Read the model definition and answer for the solid it produces. Units are mm, in the model's axes. A direction names the side the tool comes from. Round coordinates to 2 decimals unless told otherwise and drop trailing zeros. Write each loop counter-clockwise with the first axis right and the second up, starting at its lowest first coordinate (ties: lowest second). Pieces come first, ordered by that corner, then holes.
from build123d import *

# Parameters (mm, degrees)
F1_DEPTH       = 12.5
F2_R           = 5
F4_D           = 5
F4_DEPTH       = 20
F4_CBORE_D     = 10
F4_CBORE_DEPTH = 5
F4_TIP         = 1.5021515476
F6_D           = 4
F6_CSINK_D     = 10
F6_CSINK_ANGLE = 90


with BuildPart() as f1:
    # F0 (on Top) → F1 (new body, symmetric)
    with BuildSketch(Plane.XY):
        with BuildLine():
            Line((75, 27.5), (-75, 27.5))
            Line((-75, 27.5), (-75, -27.5))
            Line((-75, -27.5), (-25, -27.5))
            ThreePointArc((-25, -27.5), (0, -2.5), (25, -27.5))
            Line((25, -27.5), (75, -27.5))
            Line((75, -27.5), (75, 27.5))
        make_face()
    extrude(amount=F1_DEPTH, both=True)

    # F2
    f2_edges = [f1.edges().sort_by_distance(p)[0] for p in [
        (75, 27.5, 0),
        (-75, 27.5, 0),
        (-75, -27.5, 0),
        (75, -27.5, 0),
    ]]
    fillet(f2_edges, radius=F2_R)

    # F4
    with Locations(Plane.XY.offset(12.5)):
        with Locations((-55, 7.5), (55, 7.5)):
            CounterBoreHole(F4_D / 2, F4_CBORE_D / 2, F4_CBORE_DEPTH, depth=F4_DEPTH)
            with Locations((0, 0, -(F4_DEPTH + F4_TIP / 2))):  # 118° drill point
                Cone(0, F4_D / 2, F4_TIP, mode=Mode.SUBTRACT)

    # F6 (through all)
    with Locations(Plane(origin=(0, 27.5, 0), x_dir=(-1, 0, 0), z_dir=(0, 1, 0))):
        with Locations((0, 0)):
            CounterSinkHole(F6_D / 2, F6_CSINK_D / 2, counter_sink_angle=F6_CSINK_ANGLE)


solid = f1.part
Q1. Determine the mould class of faces 1 (the conical face through (-0.465, 24.646, -2.095)), 2 (the cylindrical face through (73.57, -26, -0.18)), 3 (the cylindrical face through (-57.31, 6.54, -0.11)), 4 (the cylindrical face through (-73.5, -26.07, 0.18)) for opening direction X: pulls with the +X half, pulls with the -X half, needs draft (parallel to the pull), parting line crosses it, or undercut.
Verdict:
face 1: undercut
face 2: pulls with the +X half
face 3: undercut
face 4: pulls with the -X half
Q2. Section A-A (z = 0) is taken. Determine the outline of the cut face in (x, y), then the cut area to 3 significant figures.
Verdict:
outline: (-75, -22.5) arc R5 ccw to (-70, -27.5) - (-25, -27.5) arc R25 cw to (-2, -2.58) - (-2, 24.5) - (-5, 27.5) - (-70, 27.5) arc R5 ccw to (-75, 22.5) - close; (2, -2.58) arc R25 cw to (25, -27.5) - (70, -27.5) arc R5 ccw to (75, -22.5) - (75, 22.5) arc R5 ccw to (70, 27.5) - (5, 27.5) - (2, 24.5) - close; hole circle Ø5 at (-55, 7.5); hole circle Ø5 at (55, 7.5)
area: 7,080 mm2
Q3. Straight lines are drawn through the part: probe 1 along X at (y, z) = (7.5, -3.75); probe 2 along X at (y, z) = (11.75, 0); probe 3 along X at (y, z) = (7.5, -1). For each, find the intervals that lie inside material, in ascending order.
Verdict:
probe 1: x = -75 to -57.5, -52.5 to 52.5, 57.5 to 75
probe 2: x = -75 to -2, 2 to 75
probe 3: x = -75 to -57.5, -52.5 to -1.73, 1.73 to 52.5, 57.5 to 75
Q4. Section B-B (z = 9.5) is taken. Determine the outline of the cut face in (x, y), then the cut area to 3 significant figures.
Verdict:
outline: (-75, -22.5) arc R5 ccw to (-70, -27.5) - (-25, -27.5) arc R25 cw to (25, -27.5) - (70, -27.5) arc R5 ccw to (75, -22.5) - (75, 22.5) arc R5 ccw to (70, 27.5) - (-70, 27.5) arc R5 ccw to (-75, 22.5) - close; hole circle Ø10 at (-55, 7.5); hole circle Ø10 at (55, 7.5)
area: 7,090 mm2
Q5. Flat-ended cylindrical pins translate along their axes: pin 1 Ø11 at (x, y) = (55, 9) entering from +Z; pin 2 Ø4 at (x, z) = (6, 2.5) entering from -Y; pin 3 Ø5 at (x, y) = (-54, 9) entering from +Z; pin 4 Ø4.5 at (x, z) = (0, 0) entering from -Y. Find the tip coordinate at first contact, or state that the pin passes through.
Verdict:
pin 1: stops at z = 12.5
pin 2: stops at y = -3.81
pin 3: stops at z = 7.5
pin 4: stops at y = -2.6
Q6. Which of the six approach directions +Z, -Z, +X, -X, +Y, -Y give full straight-line access (tool end or side, diameter ignored) to faces 5 (the cylindrical face through (-59.995, 7.72, 10.035)), 6 (the flat face through (47, -27.5, 0))?
Verdict:
face 5: +Z
face 6: +Z, -Z, +X, -X, -Y
